from build123d import *

# Parameters (mm, degrees)
BOSS_EXTRUDE1_DEPTH = 45
SKETCH2_W           = 29
SKETCH2_H           = 38
SKETCH3_W           = 78
SKETCH3_H           = 90
SKETCH3_W_2         = 58
SKETCH3_H_2         = 38
BOSS_EXTRUDE2_DEPTH = 6


with BuildPart() as part:
    # Sketch1 → Boss-Extrude1 (new, symmetric)
    with BuildSketch(Plane(origin=(0, 0, 0), x_dir=(-1, 0, 0), z_dir=(0, 1, 0))):
        Polygon((39, 0), (29, 0), (-29, 0), (-39, 0), (-39, -35), (39, -35), align=None)
    extrude(amount=BOSS_EXTRUDE1_DEPTH, both=True)

    # Sketch2 → Cut-Revolve4 (revolve, cut)
    with BuildSketch(Plane.XY):
        with Locations((-14.5, -21)):
            Rectangle(SKETCH2_W, SKETCH2_H)
        with Locations((-14.5, 21)):
            Rectangle(SKETCH2_W, SKETCH2_H)
    revolve(axis=Axis((0, 45, 0), (0, -1, 0)), mode=Mode.SUBTRACT)

    # Sketch3 → Boss-Extrude2 (add)
    with BuildSketch(Plane.XY):
        Rectangle(SKETCH3_W, SKETCH3_H)
        with Locations((0, -21)):
            Rectangle(SKETCH3_W_2, SKETCH3_H_2, mode=Mode.SUBTRACT)
        with Locations((0, 21)):
            Rectangle(SKETCH3_W_2, SKETCH3_H_2, mode=Mode.SUBTRACT)
    extrude(amount=BOSS_EXTRUDE2_DEPTH)


solid = part.part
The listing builds one solid part. Answer for the finished solid, in the listing's coordinates (mm). A direction names the side the tool comes from. Coordinates: 2 decimals unless noted, no trailing zeros. Loops run counter-clockwise (first coordinate to the right, second up) from the corner with the lowest first, then second, coordinate; pieces in that order, holes last.
1) Find the intervals of material crossed by L1, parallel to Y at x = 9.5, z = -10; L2, parallel to X at y = 29, z = 2; L3, parallel to X at y = -7.5, z = -11.5, in increasing order.
2) A tool of negligible diameter and unlimited length cuts with its end or side. For faces 1 (the face through (29, -21, 3)), 2 (the face through (-1, 45, -15)), from which of +Z, -Z, +X, -X, +Y, -Y can it reach the whole face along a straight path? Write none if from no direction.
3) Flat-ended cylindrical pins translate along their axes: pin 1 Ø1 at (x, y) = (-11, 26.5) entering from +Z; pin 2 Ø6 at (x, y) = (-23.5, 10.5) entering from +Z. Find the tip coordinate at first contact, or state that the pin passes through.
4) Find section B-B on y = -26. Write down the section's boundary in (x, z), then the cut area to 3 significant figures.
5) Find section D-D on z = -3. Write down the section's boundary in (x, y), then the cut area to 3 significant figures.
6) Find section C-C on z = -19.5. Write down the section's boundary in (x, y).
7) Determine the mould class of faces 3 (the face through (-39, -1, -15)), 4 (the face through (39, -1, -15)), 5 (the face through (-1, -45, -15)), 6 (the face through (29, 21, 3)) for opening direction X: pulls with the +X half, pulls with the -X half, needs draft (parallel to the pull), parting line crosses it, or undercut.
8) Find section A-A on x = 0. Write down the section's boundary in (y, z).
Values:
1. L1: y = -45 to -40, -2 to 2, 40 to 45
1. L2: x = -39 to -29, 29 to 39
1. L3: x = -39 to -26.62, 26.62 to 39
2. face 1: +Z
2. face 2: +Z, -Z, +X, -X, +Y
3. pin 1: stops at z = -26.62
3. pin 2: stops at z = -11.78
4. outline: (-39, -35) - (39, -35) - (39, 6) - (29, 6) - (29, 0) arc R29 cw to (-29, 0) - (-29, 6) - (-39, 6) - close
4. area: 1,530 mm2
5. outline: (-39, -45) - (39, -45) - (39, 45) - (-39, 45) - close; hole (-28.84, -40) - (28.84, -40) - (28.84, -2) - (-28.84, -2) - close; hole (-28.84, 2) - (28.84, 2) - (28.84, 40) - (-28.84, 40) - close
5. area: 2,640 mm2
6. outline: (-39, -45) - (39, -45) - (39, 45) - (-39, 45) - close; hole (-21.47, -40) - (21.47, -40) - (21.47, -2) - (-21.47, -2) - close; hole (-21.47, 2) - (21.47, 2) - (21.47, 40) - (-21.47, 40) - close
7. face 3: pulls with the -X half
7. face 4: pulls with the +X half
7. face 5: needs draft
7. face 6: undercut
8. outline: (-45, -35) - (45, -35) - (45, 6) - (40, 6) - (40, -29) - (2, -29) - (2, 6) - (-2, 6) - (-2, -29) - (-40, -29) - (-40, 6) - (-45, 6) - close
